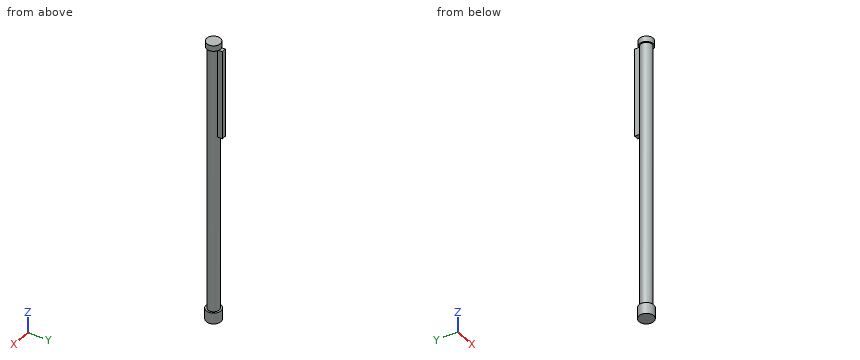
```python
from build123d import *

# Parameters (mm, degrees)
SKETCH1_R           = 3.175
BOSS_EXTRUDE1_DEPTH = 152.4
SKETCH2_W           = 2.54
SKETCH2_H           = 5.08
BOSS_EXTRUDE4_DEPTH = 50.8
SKETCH3_R           = 4.162568093
BOSS_EXTRUDE5_DEPTH = 6.35
SKETCH4_R           = 3.861049132
BOSS_EXTRUDE6_DEPTH = 3.175


with BuildPart() as part:
    # Sketch1 → Boss-Extrude1 (new body)
    with BuildSketch(Plane.XY):
        with Locations(Location((0, 0, 0), (0, 0, 180))):
            Circle(SKETCH1_R)
    extrude(amount=BOSS_EXTRUDE1_DEPTH)

    # Sketch2 → Boss-Extrude4 (add)
    with BuildSketch(Plane.XY.offset(152.4)):
        with Locations((0, 3.175)):
            Rectangle(SKETCH2_W, SKETCH2_H)
    extrude(amount=-BOSS_EXTRUDE4_DEPTH)

    # Sketch3 → Boss-Extrude5 (add)
    with BuildSketch(Plane(origin=(0, 0, 0), x_dir=(-1, 0, 0), z_dir=(0, 0, -1))):
        Circle(SKETCH3_R)
    extrude(amount=BOSS_EXTRUDE5_DEPTH)

    # Sketch4 → Boss-Extrude6 (add)
    with BuildSketch(Plane.XY.offset(152.4)):
        with Locations(Location((0, 0, 0), (0, 0, 109.203609726))):
            Circle(SKETCH4_R)
    extrude(amount=BOSS_EXTRUDE6_DEPTH)


solid = part.part
```
Input: part model. Units: mm. Frame: model coordinates. Coordinates: 2 decimals unless noted, no trailing zeros. Loops run counter-clockwise (first coordinate to the right, second up) from the corner with the lowest first, then second, coordinate; pieces in that order, holes last. Notation, with made-up numbers: M 80.25,67 L 92.25,67 A34 cw 92.25,98 Z; hole C -40,78.25 d4. An arc over 180 degrees is marked long. Use a Markdown table: item, result. Add a question column.
1) Section C-C, the plane z = 22.5. Return the cut outline in (x, y) (3 decimals), plus the area to 3 significant figures.
2) Section B-B, the plane z = 141.5. Return the cut outline in (x, y) (3 decimals), plus the area to 3 significant figures.
3) Section A-A, the plane y = 0. Return the cut outline in (x, z) (3 decimals), plus the area to 3 significant figures.
4) Line query: L1, parallel to Z at x = -2.5, y = -2.25 (3 decimals); L2, parallel to X at y = 0.25, z = 136.5; L3, parallel to X at y = 3.25, z = 141.5. Output: solid intervals per line, ascending. Write a range as from..to.
5) Pin query (flat end, axial travel): P1, Ø2, axis at x = 3, z = 61, coming from the -Y side; P2, Ø1.5, axis at y = -2.5, z = 12.5, coming from the +X side; P3, Ø2, axis at y = -3, z = 113.5, coming from the -X side. Return the tip coordinate at first contact, or that it passes through.
Answer below:
| question | item | result |
|---|---|---|
| 1 | outline | C 0,0 d6.35 |
| 1 | area | 31.7 mm2 |
| 2 | outline | M -1.27,2.91 A3.175 ccw long 1.27,2.91 L 1.27,5.715 L -1.27,5.715 Z |
| 2 | area | 38.3 mm2 |
| 3 | outline | M -4.163,-6.35 L 4.163,-6.35 L 4.163,0 L 3.175,0 L 3.175,152.4 L 3.861,152.4 L 3.861,155.575 L -3.861,155.575 L -3.861,152.4 L -3.175,152.4 L -3.175,0 L -4.163,0 Z |
| 3 | area | 1,050 mm2 |
| 4 | L1 | -6.35..0, 152.4..155.575 |
| 4 | L2 | -3.17..3.17 |
| 4 | L3 | -1.27..1.27 |
| 5 | P1 | y = -2.47 |
| 5 | P2 | x = 2.65 |
| 5 | P3 | x = -2.47 |
